from build123d import *

# Parameters (mm, degrees)
SKETCH1_W           = 64.133812
SKETCH1_H           = 15.995398686
BOSS_EXTRUDE1_DEPTH = 1.75


with BuildPart() as part:
    # Sketch1 → Boss-Extrude1 (new body)
    with BuildSketch(Plane.XY):
        Rectangle(SKETCH1_W, SKETCH1_H)
        Polygon((-12.5, -2.075), (-10.35, -2.075), (-10.35, -2.575), (10.35, -2.575), (10.35, -2.075), (12.5, -2.075), (12.5, 2.075), (10.35, 2.075), (10.35, 2.575), (2, 2.575), (2, 4.175), (-2, 4.175), (-2, 2.575), (-10.35, 2.575), (-10.35, 2.075), (-12.5, 2.075), align=None, mode=Mode.SUBTRACT)
    extrude(amount=BOSS_EXTRUDE1_DEPTH)


solid = part.part
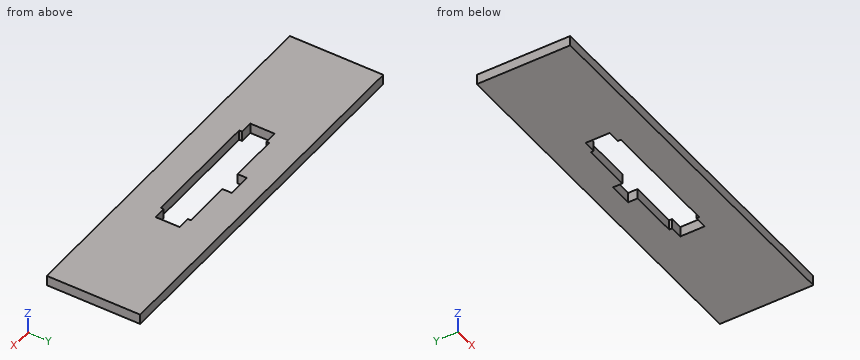
Can you work these out from the model? Positions are in its coordinate system, mm. Give positions to 0.01 mm unless a question says otherwise; leave off trailing zeros. Write each loop counter-clockwise with the first axis right and the second up, starting at its lowest first coordinate (ties: lowest second). Pieces come first, ordered by that corner, then holes. Notation, with made-up numbers: (49.25, 40) -> (107.25, 40) arc R19 cw to (107.25, 63) -> close; hole circle Ø7 at (-11.75, -21.75). An arc over 180 degrees is marked (long way). Answer as a JSON object with one key per item and string values. Group by question number.
Item 1: Suppose I cut it at A-A (y = 3.5). Please give me the cut outline in (x, z), plus the area to 3 significant figures.
Item 2: Suppose I cut it at B-B (z = 0.4). Please give me the cut outline in (x, y) (3 decimals).
Item 3: Please list where these lines run through material, in increasing order: line 1 (Y direction, x = -6, z = 0.9) (3 decimals); line 2 (X direction, y = -0.25, z = 1.45); line 3 (Y direction, x = 0, z = 1.6) (3 decimals). Write a range as [from, to].
Item 4: Suppose I cut it at C-C (x = 1). Please give me the cut outline in (y, z) (3 decimals), plus the area to 3 significant figures.
Findings:
{
 "1": {"outline": "(-32.07, 0) -> (-2, 0) -> (-2, 1.75) -> (-32.07, 1.75) -> close; (2, 0) -> (32.07, 0) -> (32.07, 1.75) -> (2, 1.75) -> close", "area": "105 mm²"},
 "2": {"outline": "(-32.067, -7.998) -> (32.067, -7.998) -> (32.067, 7.998) -> (-32.067, 7.998) -> close; hole (-12.5, -2.075) -> (-10.35, -2.075) -> (-10.35, -2.575) -> (10.35, -2.575) -> (10.35, -2.075) -> (12.5, -2.075) -> (12.5, 2.075) -> (10.35, 2.075) -> (10.35, 2.575) -> (2, 2.575) -> (2, 4.175) -> (-2, 4.175) -> (-2, 2.575) -> (-10.35, 2.575) -> (-10.35, 2.075) -> (-12.5, 2.075) -> close"},
 "3": {"line 1": "y = [-7.998, -2.575], [2.575, 7.998]", "line 2": "x = [-32.07, -12.5], [12.5, 32.07]", "line 3": "y = [-7.998, -2.575], [4.175, 7.998]"},
 "4": {"outline": "(-7.998, 0) -> (-2.575, 0) -> (-2.575, 1.75) -> (-7.998, 1.75) -> close; (4.175, 0) -> (7.998, 0) -> (7.998, 1.75) -> (4.175, 1.75) -> close", "area": "16.2 mm²"}
}
